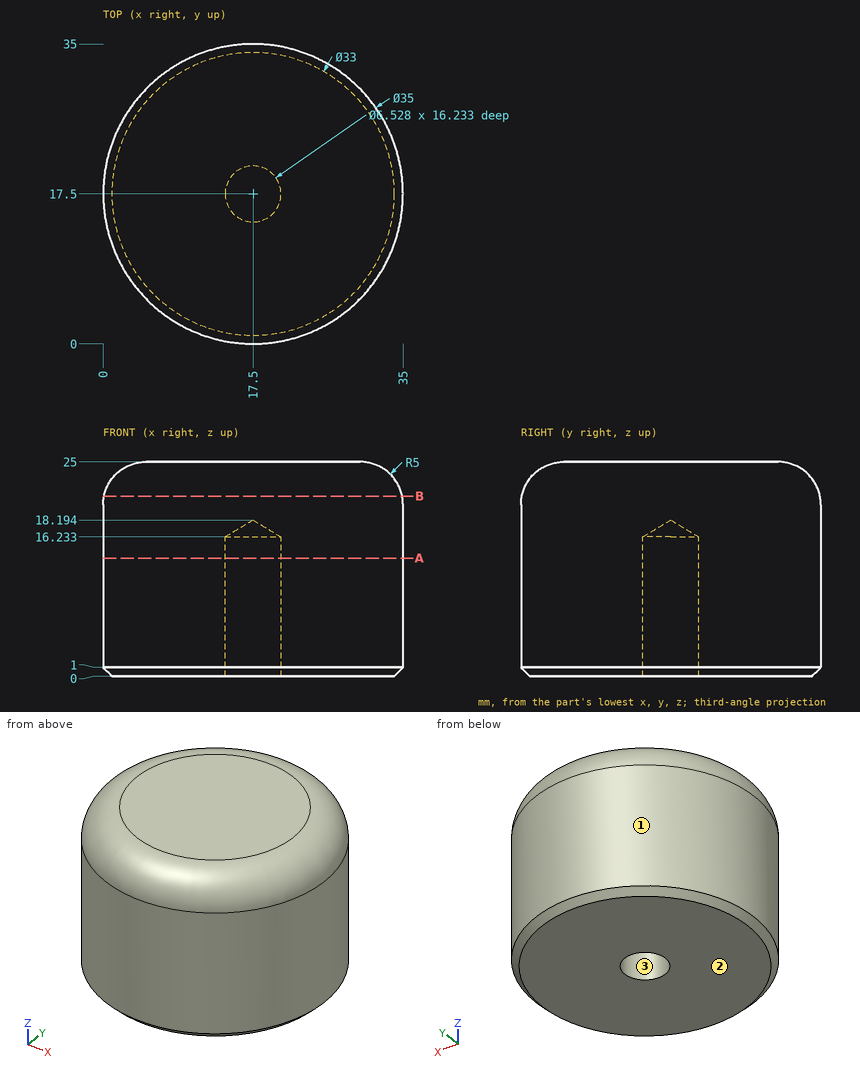
Drawing for the job (mm, zero at the part's lowest x, y, z). Round coordinates to 2 decimals unless told otherwise and drop trailing zeros. Write each loop counter-clockwise with the first axis right and the second up, starting at its lowest first coordinate (ties: lowest second). Pieces come first, ordered by that corner, then holes. Notation, with made-up numbers: (-19, -7.75) - (31, -7.75) arc R19 ccw to (31, -2.75) - close; hole circle Ø8 at (43, 26.25). An arc over 180 degrees is marked (long way). Write item = value, one per line. Start each with the question number.
Q1. Probe L1, parallel to Y at x = 17.5, z = 6.25; L2, parallel to X at y = 19, z = 2 (1 decimal); L3, parallel to Z at x = 30, y = 15.5. List the from-to ranges inside material, lowest first. Write a range as from..to.
Q2. Mould opens along Y. For the marked faces 1, 2 and 3 say: pulls with the +Y half, pulls with the -Y half, needs draft (parallel to the pull), parting line crosses it, or undercut.
Q3. Band-saw the part on B-B (z = 21). Give the cut face in (x, y).
Q4. Drop flat-ended pins along their axis: pin 1 (2 mm diameter, centred on y = 8, z = 18, fed in from +X); pin 2 (2 mm diameter, centred on y = 28, z = 18, fed in from +X); pin 3 (2 mm diameter, centred on y = 16, z = 10.5, fed in from -X). Give the stop position or say it passes through.
Q5. Band-saw the part on A-A (z = 13.75). Give the cut face in (x, y), then the cut area to 3 significant figures.
Answers below:
q1.L1 = 0..14.24, 20.76..35
q1.L2 = 0.1..14.6, 20.4..34.9
q1.L3 = 0..25
q2.face_1 = parting line crosses it
q2.face_2 = needs draft
q2.face_3 = undercut
q3.outline = circle Ø34.8 at (17.5, 17.5)
q4.pin_1 = 32.8
q4.pin_2 = 32.2
q4.pin_3 = 0.01
q5.outline = circle Ø35 at (17.5, 17.5); hole circle Ø6.53 at (17.5, 17.5)
q5.area = 929 mm2
